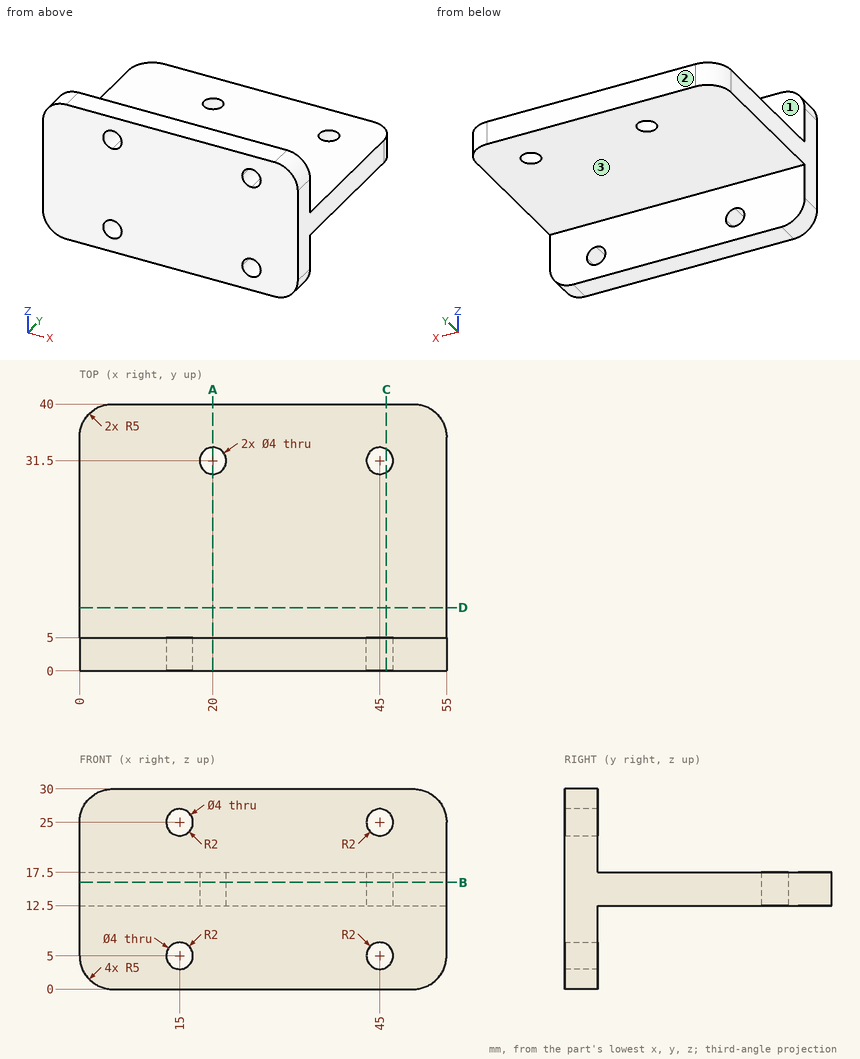
Study the drawing (mm; zero at the part's minimum x, y, z) and answer. A direction names the side the tool comes from. Coordinates: 2 decimals unless noted, no trailing zeros. Order: outer loops, then holes, each group sorted by start corner. A loop starts at its lowest first (then second) coordinate and runs counter-clockwise, first axis right, second up. Notation, with made-up numbers: (36.25, -8.75) -> (78.25, -8.75) arc R30 cw to (78.25, 22.25) -> close; hole circle Ø4 at (22.25, 33.25). An arc over 180 degrees is marked (long way). Answer in a Markdown table with one row per item. Add a question column.
Item 1: Find section D-D (y = 9.5). Write down the section's boundary in (x, z).
Item 2: Find section C-C (x = 46). Write down the section's boundary in (y, z), then the cut area to 3 significant figures.
Item 3: Find the intervals of material crossed by L1, parallel to Z at x = 15, y = 1.75; L2, parallel to X at y = 2.85, z = 25; L3, parallel to Y at x = 45, z = 14.2, in increasing order. Write a range as from..to.
Item 4: Which of the six approach directions +Z, -Z, +X, -X, +Y, -Y give full straight-line access (tool end or side, diameter ignored) to the marked faces 1, 2 and 3?
Item 5: Find section A-A (x = 20). Write down the section's boundary in (y, z).
Item 6: Each of these flat-tipped pins is pushed along its axis until it touches: P1, Ø4, axis at x = 26, y = 17, coming from the -Z side; P2, Ø2.5, axis at x = 15, z = 25, coming from the -Y side; P3, Ø12, axis at x = 25, y = 33, coming from the +Z side; P4, Ø4, axis at x = 33, z = 4.5, coming from the +Y side. Where does it stop, or does it pass through?
Item 7: Find section B-B (z = 16). Write down the section's boundary in (x, y).
Result set:
| question | item | result |
|---|---|---|
| 1 | outline | (0, 12.5) -> (55, 12.5) -> (55, 17.5) -> (0, 17.5) -> close |
| 2 | outline | (0, 0) -> (5, 0) -> (5, 3.27) -> (0, 3.27) -> close; (0, 6.73) -> (5, 6.73) -> (5, 12.5) -> (29.77, 12.5) -> (29.77, 17.5) -> (5, 17.5) -> (5, 23.27) -> (0, 23.27) -> close; (0, 26.73) -> (5, 26.73) -> (5, 30) -> (0, 30) -> close; (33.23, 12.5) -> (40, 12.5) -> (40, 17.5) -> (33.23, 17.5) -> close |
| 2 | area | 273 mm² |
| 3 | L1 | z = 0..3, 7..23, 27..30 |
| 3 | L2 | x = 0..13, 17..43, 47..55 |
| 3 | L3 | y = 0..29.5, 33.5..40 |
| 4 | face 1 | +Z, +X, -X, +Y |
| 4 | face 2 | +Z, -Z, +X, -X, +Y |
| 4 | face 3 | -Z, +X, -X, +Y |
| 5 | outline | (0, 0) -> (5, 0) -> (5, 12.5) -> (29.5, 12.5) -> (29.5, 17.5) -> (5, 17.5) -> (5, 30) -> (0, 30) -> close; (33.5, 12.5) -> (40, 12.5) -> (40, 17.5) -> (33.5, 17.5) -> close |
| 6 | P1 | stops at z = 12.5 |
| 6 | P2 | passes through |
| 6 | P3 | stops at z = 17.5 |
| 6 | P4 | stops at y = 5 |
| 7 | outline | (0, 0) -> (55, 0) -> (55, 35) arc R5 ccw to (50, 40) -> (5, 40) arc R5 ccw to (0, 35) -> close; hole circle Ø4 at (20, 31.5); hole circle Ø4 at (45, 31.5) |
